Geometry: final body of the model. Coordinates: model frame, mm. Face numbers are marked on the shaded views. Give positions to 0.01 mm unless a question says otherwise; leave off trailing zeros. Loops run counter-clockwise (first coordinate to the right, second up) from the corner with the lowest first, then second, coordinate; pieces in that order, holes last. Notation, with made-up numbers: (-28, -15.5) -> (-17, -15.5) arc R23 ccw to (-17, 6.5) -> close; hole circle Ø7 at (22, -10.75). An arc over 180 degrees is marked (long way). Answer in a Markdown table with one row per item. Add a question column.
1) Section query B-B (x = 0). Return the cut outline in (y, z).
2) Line query: line 1 (Z direction, x = 0, y = 2.2); line 2 (X direction, y = 1.75, z = -3); line 3 (X direction, y = 1.85, z = -4.5). Output: solid intervals per line, ascending. Write a range as from..to.
3) Section query C-C (y = 0.75). Return the cut outline in (x, z).
4) First-contact query: P1, Ø1.5, axis at x = -2, y = 2.5, coming from the -Z side. Flat tip, straight axial feed; report the tip coordinate or a pass-through.
5) Draft query along Z for the marked faces 1, 2 and 3. Return one class per face: +Z half, -Z half, draft (parallel to the pull), parting line (faces both ways), or undercut.
6) Section query A-A (z = 0). Return the cut outline in (x, y), plus the area to 3 significant figures.
Autodesk Inventor part; units mm, degrees
ref_plane "YZ Plane" through (0, 0, 0) normal (1, 0, 0) x (0, 1, 0)
ref_plane "XZ Plane" through (0, 0, 0) normal (0, 1, 0) x (-1, 0, 0)
ref_plane "XY Plane" through (0, 0, 0) normal (0, 0, 1) x (1, 0, 0)
sketch "Sketch1" plane through (0, 0, 0) normal (0, 1, 0) x (-1, 0, 0)
  circle A0 centre (0, 0) radius 7.5
  dimension "d0" = 15
extrude "Extrusion1" add sketch "Sketch1" along normal blind 5
sketch "Sketch2" plane through (0, 5, 0) normal (0, 1, 0) x (1, 0, 0)
  point P0 (0, 0)
  point P1 (0, 0)
hole "Hole1" at (0, 5, 0) direction (0, -1, 0) diameter 10.2 end through all
chamfer "Chamfer1" distance 0.5 angle 45 4 edges at (7.5, 5, 0) (0, 5, -5.1) (0, 0, -5.1) (7.5, 0, 0)
properties part number "Case Bottom Ring"
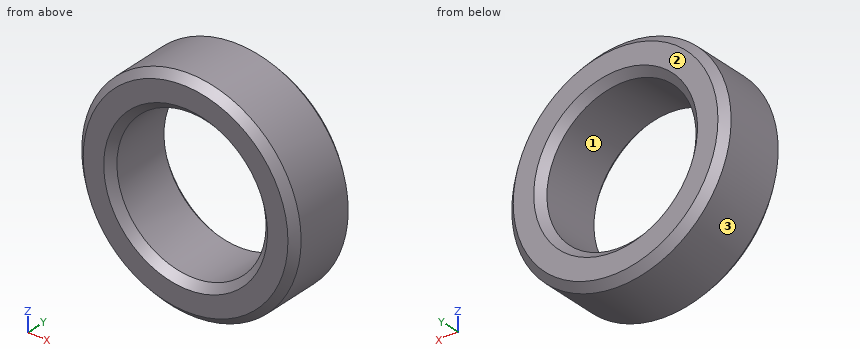
Evaluation:
| question | item | result |
|---|---|---|
| 1 | outline | (0, -7) -> (0.5, -7.5) -> (4.5, -7.5) -> (5, -7) -> (5, -5.6) -> (4.5, -5.1) -> (0.5, -5.1) -> (0, -5.6) -> close; (0, 5.6) -> (0.5, 5.1) -> (4.5, 5.1) -> (5, 5.6) -> (5, 7) -> (4.5, 7.5) -> (0.5, 7.5) -> (0, 7) -> close |
| 2 | line 1 | -7.5..-5.1, 5.1..7.5 |
| 2 | line 2 | -6.87..-4.12, 4.12..6.87 |
| 2 | line 3 | -6..-2.4, 2.4..6 |
| 3 | outline | circle Ø15 at (0, 0); hole circle Ø10.2 at (0, 0) |
| 4 | P1 | z = -7.4 |
| 5 | face 1 | undercut |
| 5 | face 2 | draft |
| 5 | face 3 | parting line |
| 6 | outline | (-7.5, 0.5) -> (-7, 0) -> (-5.6, 0) -> (-5.1, 0.5) -> (-5.1, 4.5) -> (-5.6, 5) -> (-7, 5) -> (-7.5, 4.5) -> close; (5.1, 0.5) -> (5.6, 0) -> (7, 0) -> (7.5, 0.5) -> (7.5, 4.5) -> (7, 5) -> (5.6, 5) -> (5.1, 4.5) -> close |
| 6 | area | 23.0 mm² |
